Could you check a few things on this drawing? It's one solid part, dimensions in mm from its lowest x, y, z. A direction names the side the tool comes from. Coordinates: 2 decimals unless noted, no trailing zeros. Order: outer loops, then holes, each group sorted by start corner. A loop starts at its lowest first (then second) coordinate and runs counter-clockwise, first axis right, second up. Notation, with made-up numbers: M 15,73 L 72,73 A20 cw 72,108 Z; hole C 61.25,35.25 d3. An arc over 180 degrees is marked long. One line per question, with ' | ' between items. Start each with the question number.
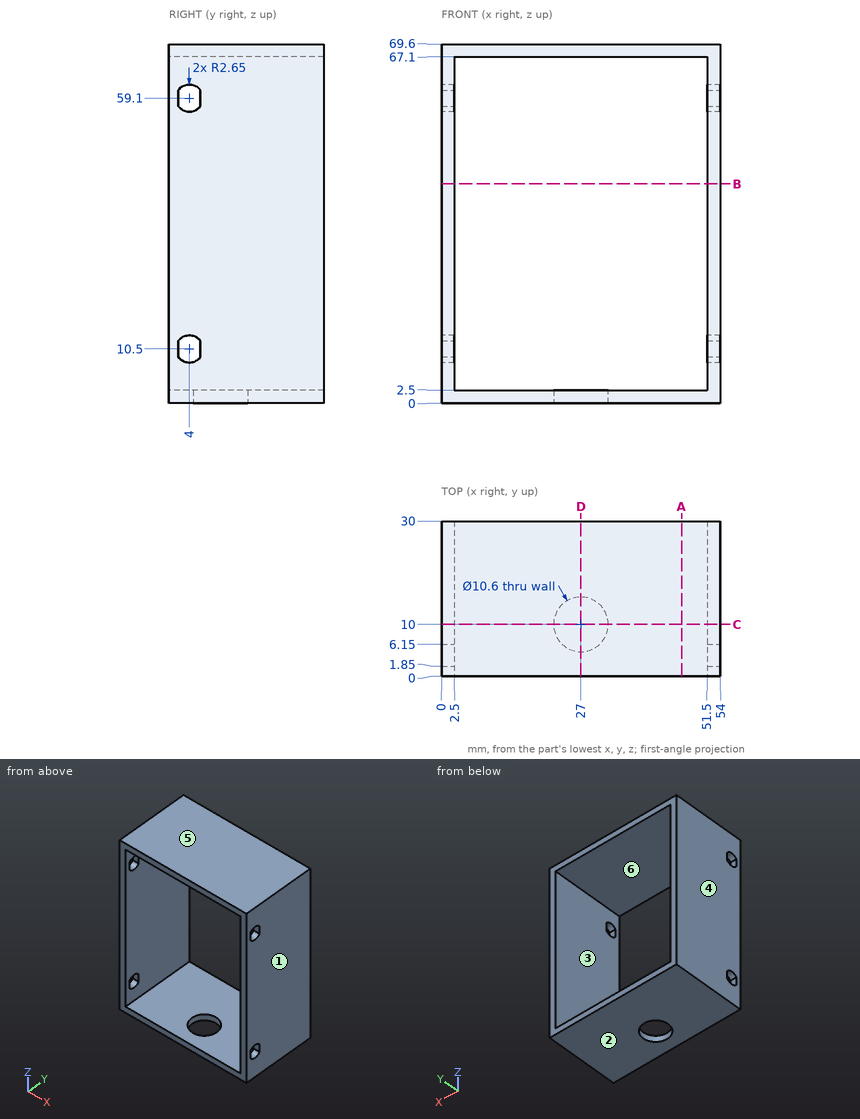
1. Imagine slicing it at C-C (y = 10). List the corners of the cut face in (x, z) for me.
2. Imagine slicing it at A-A (x = 46.5). List the corners of the cut face in (y, z) for me, then the cut area to 3 significant figures.
3. Which directions (+Z, -Z, +X, -X, +Y, -Y) give clear straight access to the entire face, cutting with the end or side of a thin tool? Please do the marked faces 5 and 6.
4. Imagine slicing it at B-B (z = 42.5). List the corners of the cut face in (x, y) for me.
5. Imagine slicing it at D-D (x = 27). List the corners of the cut face in (y, z) for me, then the cut area to 4 significant figures.
6. I need wall thicknesses on line 1 (Z direction, x = 46, y = 23.75); line 2 (X direction, y = 12, z = 64.5); line 3 (Y direction, x = 27, z = 1.9). Which ranges of each line are inside material? Lowest first, please.
7. We'd pull the mould along X, two halves only. Please class the marked faces 1, 2, 3 and 4: released by +X, released by -X, zero draft, split by the parting line, or undercut.
8. Will this pin go through, and if not, where does the flat tip stop? pin 1 (0.8 mm diameter, centred on x = 53, z = 59, fed in from -Y).
Entries:
1) outline: M 0,0 L 21.7,0 L 21.7,2.5 L 2.5,2.5 L 2.5,67.1 L 51.5,67.1 L 51.5,2.5 L 32.3,2.5 L 32.3,0 L 54,0 L 54,69.6 L 0,69.6 Z
2) outline: M 0,0 L 30,0 L 30,2.5 L 0,2.5 Z; M 0,67.1 L 30,67.1 L 30,69.6 L 0,69.6 Z | area: 150 mm²
3) face 5: +Z, +X, -X, +Y, -Y | face 6: +Y, -Y
4) outline: M 0,0 L 2.5,0 L 2.5,30 L 0,30 Z; M 51.5,0 L 54,0 L 54,30 L 51.5,30 Z
5) outline: M 0,0 L 4.7,0 L 4.7,2.5 L 0,2.5 Z; M 0,67.1 L 30,67.1 L 30,69.6 L 0,69.6 Z; M 15.3,0 L 30,0 L 30,2.5 L 15.3,2.5 Z | area: 123.5 mm²
6) line 1: 0 to 2.5, 67.1 to 69.6 | line 2: 0 to 2.5, 51.5 to 54 | line 3: 0 to 4.7, 15.3 to 30
7) face 1: released by +X | face 2: zero draft | face 3: undercut | face 4: released by -X
8) pin 1: y = 0
